The figure shows three views and two pictorial views of one solid part (mm, origin at its lowest corner). Answer the questions. Coordinates: 2 decimals unless noted, no trailing zeros. Loops run counter-clockwise (first coordinate to the right, second up) from the corner with the lowest first, then second, coordinate; pieces in that order, holes last. Notation, with made-up numbers: (67, -8) - (121, -8) arc R19 ccw to (121, 7) - close; hole circle Ø8 at (44.25, 19.5). An arc over 180 degrees is marked (long way). Write each question's results on one line, items separated by ' | '. Start each with the question number.
Item 1: Section A-A, the plane x = 27 is taken. Write down the section's boundary in (y, z).
Item 2: Section B-B, the plane z = 2.1 is taken. Write down the section's boundary in (x, y).
Item 3: Consider probe 1 along X at (y, z) = (2.5, 0.85); probe 2 along Y at (x, z) = (4, 2.6); probe 3 along X at (y, z) = (4.75, 2). Determine where each line is inside the solid, lowest interval first. Write a range as [from, to].
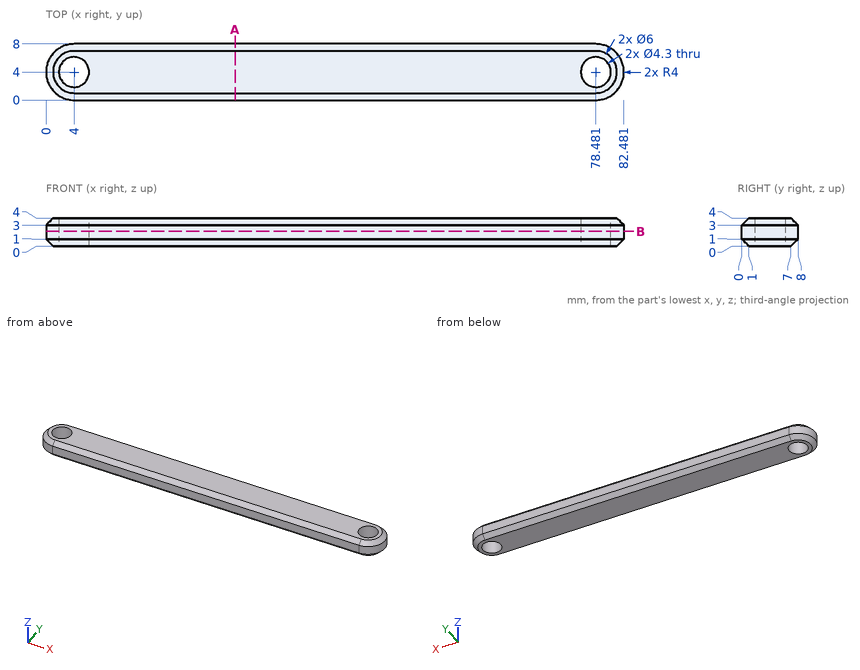
Answer key:
1) outline: (0, 1) - (1, 0) - (7, 0) - (8, 1) - (8, 3) - (7, 4) - (1, 4) - (0, 3) - close
2) outline: (4, 0) - (78.48, 0) arc R4 ccw to (78.48, 8) - (4, 8) arc R4 ccw to start; hole circle Ø4.3 at (4, 4); hole circle Ø4.3 at (78.48, 4)
3) probe 1: x = [0.45, 2.46], [5.54, 76.94], [80.02, 82.03] | probe 2: y = [0, 1.85], [6.15, 8] | probe 3: x = [0.07, 1.99], [6.01, 76.47], [80.5, 82.41]
